Geometry: final body of the model. Coordinates: model frame, mm. A direction names the side the tool comes from. Give positions to 0.01 mm unless a question says otherwise; leave off trailing zeros. Loops run counter-clockwise (first coordinate to the right, second up) from the corner with the lowest first, then second, coordinate; pieces in that order, holes last. Notation, with made-up numbers: (-4, 5.5) - (46, 5.5) arc R19 cw to (46, 28.5) - close; hole circle Ø8 at (1, 87.5). An arc over 180 degrees is marked (long way). Use CSV: the item, a comma, the result in double quotes. Start each with the question number.
```python
from build123d import *

# Parameters (mm, degrees)
SKETCH1_W           = 68
SKETCH1_H           = 68
BOSS_EXTRUDE1_DEPTH = 10
BOSS_EXTRUDE2_DEPTH = 3
BOSS_EXTRUDE3_DEPTH = 11
BOSS_EXTRUDE4_START = 3
BOSS_EXTRUDE4_DEPTH = 3
BOSS_EXTRUDE5_START = 11
BOSS_EXTRUDE5_DEPTH = 11
SKETCH6_W           = 42.5
SKETCH6_H           = 42.5
CUT_EXTRUDE1_DEPTH  = 3
SKETCH8_R           = 1.5
CUT_EXTRUDE2_DEPTH  = 15
SKETCH9_W           = 10
SKETCH9_H           = 20
BOSS_EXTRUDE6_DEPTH = 20
SKETCH10_R          = 1.5
CUT_EXTRUDE3_DEPTH  = 10
SKETCH11_R          = 1
CUT_EXTRUDE4_DEPTH  = 20
SKETCH13_W          = 7
SKETCH13_H          = 16
BOSS_EXTRUDE7_DEPTH = 40
CUT_EXTRUDE5_DEPTH  = 10
BOSS_EXTRUDE8_START = -7
BOSS_EXTRUDE8_DEPTH = 7
SKETCH17_W          = 10
SKETCH17_H          = 13.1
CUT_EXTRUDE6_DEPTH  = 10
SKETCH18_R          = 1.5
CUT_EXTRUDE7_DEPTH  = 30


with BuildPart() as part:
    # Sketch1 → Boss-Extrude1 (new body)
    with BuildSketch(Plane.XY):
        with Locations((-34, -34)):
            Rectangle(SKETCH1_W, SKETCH1_H)
    extrude(amount=BOSS_EXTRUDE1_DEPTH)

    # Sketch2 → Boss-Extrude2 (add)
    with BuildSketch(Plane.ZY.offset(68)):
        with BuildLine():
            Line((10, -19.354101966), (10, -12.645898034))
            ThreePointArc((10, -12.645898034), (5.5, -16), (10, -19.354101966))
        make_face()
        with BuildLine():
            Line((10, -55.354101966), (10, -48.645898034))
            ThreePointArc((10, -48.645898034), (5.5, -52), (10, -55.354101966))
        make_face()
    extrude(amount=BOSS_EXTRUDE2_DEPTH)

    # Sketch3 → Boss-Extrude3 (add)
    with BuildSketch(Plane.ZY.offset(71)):
        with BuildLine():
            ThreePointArc((10, -49.984435563), (6.75, -52), (10, -54.015564437))
            Line((10, -54.015564437), (10, -49.984435563))
        make_face()
        with BuildLine():
            ThreePointArc((10, -13.984435563), (6.75, -16), (10, -18.015564437))
            Line((10, -18.015564437), (10, -13.984435563))
        make_face()
    extrude(amount=BOSS_EXTRUDE3_DEPTH)

    # Sketch4 → Boss-Extrude4 (add)
    with BuildSketch(Plane(origin=(0, 0, 0), x_dir=(0, 0, -1), z_dir=(1, 0, 0)).offset(BOSS_EXTRUDE4_START)):
        with BuildLine():
            ThreePointArc((-5.5, -16), (-6.908349934, -13.19375696), (-10, -12.645898034))
            Line((-10, -12.645898034), (-10, -19.354101966))
            ThreePointArc((-10, -19.354101966), (-6.908349934, -18.80624304), (-5.5, -16))
        make_face()
        with BuildLine():
            ThreePointArc((-5.5, -52), (-6.908349934, -49.19375696), (-10, -48.645898034))
            Line((-10, -48.645898034), (-10, -55.354101966))
            ThreePointArc((-10, -55.354101966), (-6.908349934, -54.80624304), (-5.5, -52))
        make_face()
    extrude(amount=-BOSS_EXTRUDE4_DEPTH)

    # Sketch5 → Boss-Extrude5 (add)
    with BuildSketch(Plane(origin=(3, 0, 0), x_dir=(0, 0, -1), z_dir=(1, 0, 0)).offset(BOSS_EXTRUDE5_START)):
        with BuildLine():
            ThreePointArc((-6.75, -16), (-7.814145877, -14.087867682), (-10, -13.984435563))
            Line((-10, -13.984435563), (-10, -18.015564437))
            ThreePointArc((-10, -18.015564437), (-7.814145877, -17.912132318), (-6.75, -16))
        make_face()
        with BuildLine():
            ThreePointArc((-6.75, -52), (-7.814145877, -50.087867682), (-10, -49.984435563))
            Line((-10, -49.984435563), (-10, -54.015564437))
            ThreePointArc((-10, -54.015564437), (-7.814145877, -53.912132318), (-6.75, -52))
        make_face()
    extrude(amount=-BOSS_EXTRUDE5_DEPTH)

    # Sketch6 → Cut-Extrude1 (cut)
    with BuildSketch(Plane(origin=(0, 0, 0), x_dir=(-1, 0, 0), z_dir=(0, 0, -1))):
        with Locations((34, -34)):
            Rectangle(SKETCH6_W, SKETCH6_H)
    extrude(amount=-CUT_EXTRUDE1_DEPTH, mode=Mode.SUBTRACT)

    # Sketch8 → Cut-Extrude2 (cut)
    with BuildSketch(Plane(origin=(0, 0, 0), x_dir=(-1, 0, 0), z_dir=(0, 0, -1))):
        with Locations((17.75, -4.75)):
            Circle(SKETCH8_R)
        with Locations((50.25, -4.75)):
            Circle(SKETCH8_R)
        with Locations((50.25, -63.25)):
            Circle(SKETCH8_R)
        with Locations((17.75, -63.25)):
            Circle(SKETCH8_R)
    extrude(amount=-CUT_EXTRUDE2_DEPTH, mode=Mode.SUBTRACT)

    # Sketch9 → Boss-Extrude6 (add)
    with BuildSketch(Plane(origin=(0, 0, 0), x_dir=(-1, 0, 0), z_dir=(0, 0, -1))):
        with Locations((5, -34)):
            Rectangle(SKETCH9_W, SKETCH9_H)
    extrude(amount=BOSS_EXTRUDE6_DEPTH)

    # Sketch10 → Cut-Extrude3 (cut)
    with BuildSketch(Plane(origin=(0, 0, 0), x_dir=(-1, 0, 0), z_dir=(0, 0, -1))):
        with Locations((7.75, -34)):
            Circle(SKETCH10_R)
        with Locations((7.75, -78)):
            Circle(SKETCH10_R)
    extrude(amount=-CUT_EXTRUDE3_DEPTH, mode=Mode.SUBTRACT)

    # Sketch11 → Cut-Extrude4 (cut)
    with BuildSketch(Plane.XY.offset(10)):
        with Locations((-66, -52)):
            Circle(SKETCH11_R)
        with Locations(Location((-66, -16, 0), (0, 0, 180))):
            Circle(SKETCH11_R)
        with Locations(Location((-2, -52, 0), (0, 0, 180))):
            Circle(SKETCH11_R)
        with Locations((-2, -16)):
            Circle(SKETCH11_R)
    extrude(amount=-CUT_EXTRUDE4_DEPTH, mode=Mode.SUBTRACT)

    # Sketch13 → Boss-Extrude7 (add)
    with BuildSketch(Plane(origin=(0, 0, 0), x_dir=(-1, 0, 0), z_dir=(0, 0, -1))):
        with Locations((62.5, -34)):
            Rectangle(SKETCH13_W, SKETCH13_H)
    extrude(amount=BOSS_EXTRUDE7_DEPTH)

    # Sketch15 → Cut-Extrude5 (cut)
    with BuildSketch(Plane.ZY.offset(66)):
        Polygon((-40, -32), (-31, -32), (-33, -30), (-40, -30), align=None)
        Polygon((-40, -38), (-40, -36), (-31, -36), (-33, -38), align=None)
    extrude(amount=-CUT_EXTRUDE5_DEPTH, mode=Mode.SUBTRACT)

    # Sketch16 → Boss-Extrude8 (add)
    with BuildSketch(Plane.ZY.offset(66).offset(BOSS_EXTRUDE8_START)):
        Polygon((0, -26), (-40, -26), (0, -21), align=None)
        Polygon((-40, -42), (0, -47), (0, -42), align=None)
    extrude(amount=BOSS_EXTRUDE8_DEPTH)

    # Sketch17 → Cut-Extrude6 (cut)
    with BuildSketch(Plane(origin=(0, 0, -20), x_dir=(-1, 0, 0), z_dir=(0, 0, -1))):
        with Locations((5, -34)):
            Rectangle(SKETCH17_W, SKETCH17_H)
    extrude(amount=-CUT_EXTRUDE6_DEPTH, mode=Mode.SUBTRACT)

    # Sketch18 → Cut-Extrude7 (cut)
    with BuildSketch(Plane(origin=(0, -44, 0), x_dir=(-1, 0, 0), z_dir=(0, -1, 0))):
        with Locations(Location((5, 15, 0), (0, 0, 180))):
            Circle(SKETCH18_R)
    extrude(amount=-CUT_EXTRUDE7_DEPTH, mode=Mode.SUBTRACT)


solid = part.part
```
Item 1: Section B-B (z = 1.5). Give the number of separate pieces and of enclosed holes in the cut face, plus the area to 3 significant figures.
Item 2: Ray query, probe 1 along Y at (x, z) = (-2, 3.5); probe 2 along Y at (x, z) = (-50.25, 6.25); probe 3 along X at (y, z) = (-4, 4). Return the intervals inside material, ascending.
Item 3: Section D-D (y = -34). Output: boundary loops of the cut face in (x, z), plus the area to 4 significant figures.
Item 4: Mould query, pull axis Y, two halves, no side actions, for faces 1 (the flat face through (-82, -16, 9)), 2 (the flat face through (-62.451, -23.535, -20.28)), 3 (the flat face through (-68, -34, 5)). Classes: pulls with the +Y half, pulls with the -Y half, needs draft (parallel to the pull), parting line crosses it, or undercut.
Item 5: Section C-C (x = -35.5). Output: boundary loops of the cut face in (y, z), plus the area to 4 significant figures.
Item 6: Reachability of faces 4 (the flat face through (-5, -34, -10)), 5 (the flat face through (-10, -34, -8)), 6 (the flat face through (-66, -34, -15)), 7 (the cylindrical face through (-76.42, -51.94, 6.75)), 8 (the flat face through (-34, -11, 0)) from +Z, -Z, +X, -X, +Y, -Y: full face, straight path, thin tool, end or side. Return the list, or none.
Item 7: Section A-A (z = -4). Output: boundary loops of the cut face in (x, y).
Item 8: Pin query (flat end, axial travel): pin 1 Ø10 at (x, y) = (-25.5, -30) entering from -Z; pin 2 Ø8 at (y, z) = (-32, -20) entering from -X; pin 3 Ø3 at (x, z) = (-2.5, -14.5) entering from -Y. Return the tip coordinate at first contact, or that it passes through.
Outcome:
1,separate pieces,"1"
1,enclosed holes,"10"
1,area,"2,770 mm2"
2,probe 1,"y = -68 to -53, -51 to -17, -15 to 0"
2,probe 2,"y = -68 to -64.75, -61.75 to -6.25, -3.25 to 0"
2,probe 3,"x = -68 to -51.55, -48.95 to -19.05, -16.45 to 0"
3,outline,"(-68, 0) - (-66, 0) - (-66, -40) - (-59, -40) - (-59, 0) - (-55.25, 0) - (-55.25, 3) - (-12.75, 3) - (-12.75, 0) - (-10, 0) - (-10, -10) - (0, -10) - (0, 10) - (-6.25, 10) - (-6.25, 0) - (-9.25, 0) - (-9.25, 10) - (-68, 10) - close"
3,area,"902.5 mm2"
4,face 1,"needs draft"
4,face 2,"pulls with the +Y half"
4,face 3,"undercut"
5,outline,"(-68, 0) - (-55.25, 0) - (-55.25, 3) - (-12.75, 3) - (-12.75, 0) - (0, 0) - (0, 10) - (-68, 10) - close"
5,area,"552.5 mm2"
6,face 4,"-Z, +X"
6,face 5,"-Z, +Y, -Y"
6,face 6,"-Z, -X, +Y, -Y"
6,face 7,"-X"
6,face 8,"-Z"
7,outline,"(-66, -46.5) - (-59, -46.5) - (-59, -21.5) - (-66, -21.5) - close; (-10, -44) - (0, -44) - (0, -24) - (-10, -24) - close"
8,pin 1,"stops at z = 3"
8,pin 2,"stops at x = -66"
8,pin 3,"stops at y = -44"
